Could you check a few things on this model? Use its own coordinates, in mm. A direction names the side the tool comes from. Give positions to 0.01 mm unless a question says otherwise; leave off trailing zeros. Order: outer loops, then holes, each group sorted by start corner. A loop starts at its lowest first (then second) coordinate and runs counter-clockwise, first axis right, second up.
(1) Imagine slicing it at D-D, the plane x = 30. Write out the boundary of the cut face in (y, z), then the cut area to 3 significant figures.
(2) Imagine slicing it at B-B, the plane x = 11. Write out the boundary of the cut face in (y, z).
(3) Will these pins go through, and if not, where does the flat tip stop? pin 1 (0.8 mm diameter, centred on y = 29.5, z = 9, fed in from +X); pin 2 (0.6 mm diameter, centred on y = 2.5, z = 1.5, fed in from +X); pin 3 (4 mm diameter, centred on x = 44.5, y = 11.5, fed in from +Z).
(4) On a 3-axis mill with a long thin cutter (end or side, diameter ignored), from which of +Z, -Z, +X, -X, +Y, -Y can I reach the whole of each face in a straight line? I mean faces 1 (the cylindrical face through (58.43, 28.4, 5.82)), 2 (the flat face through (37, 2, 1.7)), 3 (the cylindrical face through (0.9, 29.14, 5.18)). Say none if no direction works.
(5) Imagine slicing it at A-A, the plane x = 51.5. Write out the boundary of the cut face in (y, z), then the cut area to 3 significant figures.
(6) Imagine slicing it at C-C, the plane y = 22.25. Write out the boundary of the cut face in (x, z).
(7) If we mould it in two halves opening along Z, with no side actions, what happens to faces 4 (the cylindrical face through (53.81, 29.49, 3.39)), 5 (the flat face through (10, 28, 9)), 6 (the flat face through (30, 15, 0)), 7 (the flat face through (56, 28, 7))? For each: released by +Z, released by -Z, zero draft, split by the parting line, or undercut.
(8) If I drill on probe 1 along X at (y, z) = (26, 9.25); probe 2 along Z at (x, y) = (51.5, 29.85); probe 3 along Y at (x, z) = (19, 1.25), over which ranges is the centre line in solid material (lowest first)?
from build123d import *

# Parameters (mm, degrees)
PAD_DEPTH       = 10.5
POCKET_DEPTH    = 9.5
SKETCH002_W     = 4.6
SKETCH002_H     = 1.8
POCKET001_DEPTH = 1
SKETCH003_W     = 5
SKETCH003_H     = 1.8
POCKET002_DEPTH = 1
SKETCH004_W     = 1
SKETCH004_H     = 18
SKETCH004_W_2   = 7
SKETCH004_H_2   = 1
SKETCH004_W_3   = 6
PAD001_DEPTH    = 2
CHAMFER_SIZE    = 0.9
SKETCH005_R     = 2.5
SKETCH005_W     = 11.65
SKETCH005_H     = 3.6
POCKET003_DEPTH = 2.001
SKETCH006_W     = 6.25
SKETCH006_H     = 3.8
SKETCH006_W_2   = 5
SKETCH006_H_2   = 2.5
POCKET004_DEPTH = 1
SKETCH007_W     = 3
SKETCH007_H     = 12
SKETCH007_W_2   = 5
SKETCH007_H_2   = 2
SKETCH007_W_3   = 7
SKETCH007_H_3   = 1
SKETCH007_W_4   = 1
SKETCH007_W_5   = 2
SKETCH007_W_6   = 9
PAD002_DEPTH    = 0.7
SKETCH009_W     = 2
SKETCH009_H     = 2
PAD003_DEPTH    = 6
SKETCH010_W     = 1.7
SKETCH010_H     = 12
PAD004_DEPTH    = 1.5


with BuildPart() as part:
    # Sketch → Pad (new body)
    with BuildSketch(Plane.XY):
        with BuildLine():
            ThreePointArc((0, 3), (0.87868, 0.87868), (3, 0))
            Line((3, 0), (57, 0))
            ThreePointArc((57, 0), (59.12132, 0.87868), (60, 3))
            Line((60, 3), (60, 27))
            ThreePointArc((60, 27), (59.12132, 29.12132), (57, 30))
            Line((57, 30), (3, 30))
            ThreePointArc((3, 30), (0.87868, 29.12132), (0, 27))
            Line((0, 27), (0, 3))
        make_face()
    extrude(amount=PAD_DEPTH)

    # Sketch001 (on Face10 of Pad) → Pocket (cut)
    with BuildSketch(Plane.XY.offset(10.5)):
        with BuildLine():
            ThreePointArc((3, 29), (1.585786, 28.414214), (1, 27))
            Line((1, 3), (1, 27))
            ThreePointArc((1, 3), (1.585786, 1.585786), (3, 1))
            Line((57, 1), (3, 1))
            ThreePointArc((57, 1), (58.414214, 1.585786), (59, 3))
            Line((59, 27), (59, 3))
            ThreePointArc((59, 27), (58.414211, 28.414216), (56.999993, 29))
            Line((3, 29), (56.999993, 29))
        make_face()
    extrude(amount=-POCKET_DEPTH, mode=Mode.SUBTRACT)

    # Sketch002 → Pocket001 (cut)
    with BuildSketch(Plane.XZ):
        with Locations((7, 8.6)):
            Rectangle(SKETCH002_W, SKETCH002_H)
        with Locations((30, 8.6)):
            Rectangle(SKETCH002_W, SKETCH002_H)
        with Locations((53, 8.6)):
            Rectangle(SKETCH002_W, SKETCH002_H)
    extrude(amount=-POCKET001_DEPTH, mode=Mode.SUBTRACT)

    # Sketch003 (on Face24 of Pocket001) → Pocket002 (cut)
    with BuildSketch(Plane.XZ.offset(-29)):
        with Locations((17, 8.6)):
            Rectangle(SKETCH003_W, SKETCH003_H)
        with Locations((43, 8.6)):
            Rectangle(SKETCH003_W, SKETCH003_H)
    extrude(amount=-POCKET002_DEPTH, mode=Mode.SUBTRACT)

    # Sketch004 → Pad001 (join)
    with BuildSketch(Plane.XY.offset(9.5)):
        with Locations((1.5, 15)):
            Rectangle(SKETCH004_W, SKETCH004_H)
        with Locations((13.5, 1.5)):
            Rectangle(SKETCH004_W_2, SKETCH004_H_2)
        with Locations((40, 1.5)):
            Rectangle(SKETCH004_W_2, SKETCH004_H_2)
        with Locations((24.5, 28.5)):
            Rectangle(SKETCH004_W_2, SKETCH004_H_2)
        with Locations((50, 28.5)):
            Rectangle(SKETCH004_W_3, SKETCH004_H_2)
        with Locations((58.5, 15)):
            Rectangle(SKETCH004_W, SKETCH004_H)
        with Locations((10, 28.5)):
            Rectangle(SKETCH004_W_3, SKETCH004_H_2)
        with Locations((35.5, 28.5)):
            Rectangle(SKETCH004_W_2, SKETCH004_H_2)
    extrude(amount=-PAD001_DEPTH)

    # Chamfer
    chamfer_edges = [part.edges().sort_by_distance(p)[0] for p in [
        (40, 2, 7.5),
        (13.5, 2, 7.5),
        (58, 15, 7.5),
        (2, 15, 7.5),
        (10, 28, 7.5),
        (24.5, 28, 7.5),
        (35.5, 28, 7.5),
        (50, 28, 7.5),
    ]]
    chamfer(chamfer_edges, length=CHAMFER_SIZE)

    # Sketch005 → Pocket003 (cut, through all)
    with BuildSketch(Plane.XZ.offset(-28)):
        with Locations((51.5, 4.35)):
            Circle(SKETCH005_R)
        with Locations((15.125, 4.7)):
            Rectangle(SKETCH005_W, SKETCH005_H)
    extrude(amount=-POCKET003_DEPTH, mode=Mode.SUBTRACT)

    # Sketch006 → Pocket004 (cut)
    with BuildSketch(Plane.XZ):
        with Locations((49.5, 4.8)):
            Rectangle(SKETCH006_W, SKETCH006_H)
        with Locations((20, 5.7)):
            Rectangle(SKETCH006_W_2, SKETCH006_H_2)
    extrude(amount=-POCKET004_DEPTH, mode=Mode.SUBTRACT)

    # Sketch007 (on Face10 of Pocket004) → Pad002 (join)
    with BuildSketch(Plane.XY.offset(1)):
        with Locations((2.5, 15)):
            Rectangle(SKETCH007_W, SKETCH007_H)
        with Locations((37.5, 2)):
            Rectangle(SKETCH007_W_2, SKETCH007_H_2)
        with Locations((43.5, 28.5)):
            Rectangle(SKETCH007_W_3, SKETCH007_H_3)
        with Locations((5.5, 28)):
            Rectangle(SKETCH007_W_2, SKETCH007_H_2)
        with Locations((58.5, 15)):
            Rectangle(SKETCH007_W_4, SKETCH007_H)
        with Locations((4, 2)):
            Rectangle(SKETCH007_W_5, SKETCH007_H_2)
        with Locations((29.5, 28)):
            Rectangle(SKETCH007_W_2, SKETCH007_H_2)
        with Locations((20.5, 2)):
            Rectangle(SKETCH007_W_6, SKETCH007_H_2)
    extrude(amount=PAD002_DEPTH)

    # Sketch009 → Pad003 (join)
    with BuildSketch(Plane.XY.offset(1)):
        with Locations((47, 28)):
            Rectangle(SKETCH009_W, SKETCH009_H)
        with Locations((56, 28)):
            Rectangle(SKETCH009_W, SKETCH009_H)
    extrude(amount=PAD003_DEPTH)

    # Sketch010 (on Face111 of Pad003) → Pad004 (join)
    with BuildSketch(Plane.XY.offset(1.7)):
        with Locations((1.85, 15)):
            Rectangle(SKETCH010_W, SKETCH010_H)
    extrude(amount=PAD004_DEPTH)


solid = part.part
Answer block:
1. outline: (0, 0) - (30, 0) - (30, 10.5) - (29, 10.5) - (29, 1.7) - (27, 1.7) - (27, 1) - (1, 1) - (1, 7.7) - (0, 7.7) - close; (0, 9.5) - (1, 9.5) - (1, 10.5) - (0, 10.5) - close
1. area: 48.6 mm2
2. outline: (0, 0) - (30, 0) - (30, 2.9) - (29, 2.9) - (29, 1) - (1, 1) - (1, 7.5) - (1.1, 7.5) - (2, 8.4) - (2, 9.5) - (1, 9.5) - (1, 10.5) - (0, 10.5) - close; (28, 8.4) - (28.9, 7.5) - (29, 7.5) - (29, 6.5) - (30, 6.5) - (30, 10.5) - (29, 10.5) - (29, 9.5) - (28, 9.5) - close
3. pin 1: stops at x = 59.14
3. pin 2: stops at x = 59.99
3. pin 3: stops at z = 1
4. face 1: +Z
4. face 2: none
4. face 3: +Z, -Z, -X, +Y
5. outline: (0, 0) - (30, 0) - (30, 1.85) - (29, 1.85) - (29, 1) - (1, 1) - (1, 2.9) - (0, 2.9) - close; (0, 6.7) - (1, 6.7) - (1, 7.7) - (0, 7.7) - close; (0, 9.5) - (1, 9.5) - (1, 10.5) - (0, 10.5) - close; (28, 8.4) - (28.9, 7.5) - (29, 7.5) - (29, 6.85) - (30, 6.85) - (30, 10.5) - (29, 10.5) - (29, 9.5) - (28, 9.5) - close
5. area: 40.0 mm2
6. outline: (0, 0) - (60, 0) - (60, 10.5) - (59, 10.5) - (59, 9.5) - (58, 9.5) - (58, 8.4) - (58.9, 7.5) - (59, 7.5) - (59, 1) - (1, 1) - (1, 7.5) - (1.1, 7.5) - (2, 8.4) - (2, 9.5) - (1, 9.5) - (1, 10.5) - (0, 10.5) - close
7. face 4: undercut
7. face 5: zero draft
7. face 6: released by -Z
7. face 7: released by +Z
8. probe 1: x = 0 to 1, 59 to 60
8. probe 2: z = 0 to 1.85, 6.85 to 10.5
8. probe 3: y = 0 to 3, 29 to 30
